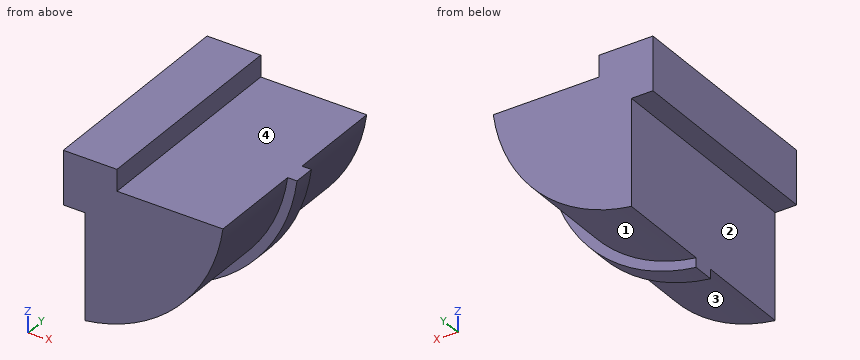
```python
from build123d import *

# Parameters (mm, degrees)
BOSS_EXTRUDE1_DEPTH = 100
BOSS_EXTRUDE2_DEPTH = 5


with BuildPart() as part:
    # Sketch2 → Boss-Extrude1 (new body)
    with BuildSketch(Plane(origin=(0, 0, 0), x_dir=(1, 0, 0), z_dir=(0, 1, 0))):
        with BuildLine():
            Line((-78.383022578, -48.650161377), (-78.383022578, -23.650161377))
            Line((-78.383022578, -23.650161377), (-68.383022578, -23.650161377))
            Line((-68.383022578, -23.650161377), (-68.383022578, 25.68018236))
            ThreePointArc((-68.383022578, 25.68018236), (-25.350013989, 4.382847212), (-4.052678842, -38.650161377))
            Line((-4.052678842, -38.650161377), (-53.383022578, -38.650161377))
            Line((-53.383022578, -38.650161377), (-53.383022578, -48.650161377))
            Line((-53.383022578, -48.650161377), (-78.383022578, -48.650161377))
        make_face()
    extrude(amount=BOSS_EXTRUDE1_DEPTH)

    # Sketch3 → Boss-Extrude2 (add, symmetric)
    with BuildSketch(Plane(origin=(0, 50, 0), x_dir=(-1, 0, 0), z_dir=(0, -1, 0))):
        with BuildLine():
            Line((68.383022578, 25.68018236), (68.383022578, 30.04988769))
            ThreePointArc((68.383022578, 30.04988769), (22.286241373, 7.446619828), (-0.317026488, -38.650161377))
            Line((-0.317026488, -38.650161377), (4.052678842, -38.650161377))
            ThreePointArc((4.052678842, -38.650161377), (25.350013989, 4.382847212), (68.383022578, 25.68018236))
        make_face()
    extrude(amount=BOSS_EXTRUDE2_DEPTH, both=True)


solid = part.part
```
Could you check a few things on this model? Use its own coordinates, in mm. Face numbers are marked on the shaded views. A direction names the side the tool comes from. Round coordinates to 2 decimals unless told otherwise and drop trailing zeros. Loops run counter-clockwise (first coordinate to the right, second up) from the corner with the lowest first, then second, coordinate; pieces in that order, holes last. Notation, with made-up numbers: M -36.5,-4.75 L 15.5,-4.75 A9 cw 15.5,6.25 Z; hole C 69.25,-19.75 d8. An arc over 180 degrees is marked long. Answer as CSV lines item,"result".
1) Imagine slicing it at D-D on x = -52. List the corners of the cut face in (y, z) for me.
From the geometry:
outline,"M 0,-21.56 L 45,-21.56 L 45,-26.17 L 55,-26.17 L 55,-21.56 L 100,-21.56 L 100,38.65 L 0,38.65 Z"
2) Which directions (+Z, -Z, +X, -X, +Y, -Y) give clear straight access to the entire face, cutting with the end or side of a thin tool? Please do the marked faces 1, 2, 3 and 4.
From the geometry:
face 1,"-Z, +X, +Y"
face 2,"-Z, -X, +Y, -Y"
face 3,"-Z, +X, -Y"
face 4,"+Z, +X, +Y, -Y"
3) Imagine slicing it at C-C on z = 40. List the corners of the cut face in (x, y) for me.
From the geometry:
outline,"M -78.38,0 L -53.38,0 L -53.38,100 L -78.38,100 Z"
4) Imagine slicing it at B-B on x = -28. List the corners of the cut face in (y, z) for me, and give its area (3 significant figures).
From the geometry:
outline,"M 0,-6.91 L 45,-6.91 L 45,-12.63 L 55,-12.63 L 55,-6.91 L 100,-6.91 L 100,38.65 L 0,38.65 Z"
area,"4,610 mm^2"
5) Imagine slicing it at A-A on y = 16.5. List the corners of the cut face in (x, z) for me, and give its area (3 significant figures).
From the geometry:
outline,"M -78.38,23.65 L -68.38,23.65 L -68.38,-25.68 A75 ccw -4.05,38.65 L -53.38,38.65 L -53.38,48.65 L -78.38,48.65 Z"
area,"3,420 mm^2"
6) For pin 1 Ø3 at (y, z) = (49.5, 0) entering from -X; pin 2 Ø12 at (x, y) = (-57, 25) entering from -Z; pin 3 Ø5 at (y, z) = (35.5, 38.5) entering from +X, each with a flat end and sliding along its axis, tell me the tip position at first contact or that it passes through.
From the geometry:
pin 1,"x = -68.38"
pin 2,"z = -24.76"
pin 3,"x = -4.05"
7) If I drill on probe 1 along Y at (x, z) = (-3.5, 33.5); probe 2 along X at (y, z) = (30, 43.5); probe 3 along X at (y, z) = (10.5, 24.5), over which ranges is the centre line in solid material (lowest first)?
From the geometry:
probe 1,"45 to 55"
probe 2,"-78.38 to -53.38"
probe 3,"-78.38 to -7.38"
